Verification items for the finished model (mm, model axes). A direction names the side the tool comes from. Round coordinates to 2 decimals unless told otherwise and drop trailing zeros. Loops run counter-clockwise (first coordinate to the right, second up) from the corner with the lowest first, then second, coordinate; pieces in that order, holes last. Notation, with made-up numbers: (80.25, 78) -> (107.25, 78) arc R3 cw to (107.25, 82) -> close; hole circle Ø1 at (-29, 52.25). An arc over 180 degrees is marked (long way). Use a Markdown table: item, result. Add a question column.
```python
from build123d import *

# Parameters (mm, degrees)
CROQUIS1_W              = 144.567109546
CROQUIS1_H              = 113.391382114
SALIENTE_EXTRUIR1_DEPTH = 200
VACIADO2_T              = -10


with BuildPart() as part:
    # Croquis1 → Saliente-Extruir1 (new body)
    with BuildSketch(Plane.XY):
        Rectangle(CROQUIS1_W, CROQUIS1_H)
    extrude(amount=SALIENTE_EXTRUIR1_DEPTH)

    # Vaciado2
    vaciado2_openings = [part.faces().sort_by_distance(p)[0] for p in [
        (0, 0, 200),
    ]]
    offset(amount=VACIADO2_T, openings=vaciado2_openings, kind=Kind.INTERSECTION)


solid = part.part
```
1) Thickness scan on line 1 (X direction, y = -22.5, z = 135); line 2 (Y direction, x = -53.5, z = 21); line 3 (Z direction, x = -29.5, y = 3.5). Record the ranges inside material, lowest first.
2) Release check for a two-part mould opening along Y. For faces 1 (the face through (-1, 56.696, 99)), 2 (the face through (-62.284, -1, 104)), 3 (the face through (72.284, -1, 99)) record: released by +Y, released by -Y, zero draft, split by the parting line, or undercut.
3) Access from +Z, -Z, +X, -X, +Y, -Y to the whole of each face (thin tool, end or side, straight path). Record for faces 4 (the face through (-1, -56.696, 99)), 5 (the face through (-1, 1, 10)).
4) Go/stop test with a flat-tipped pin: pin 1 (5 mm diameter, centred on x = 41, y = -21, fed in from +Z). Record where the tip stops, or that it passes through.
5) Sectioned sample at C-C on x = 48. Enter the section's corners in (y, z).
6) Sectioned sample at B-B on y = 29.5. Enter the section's corners in (x, z), then the cut area to 3 significant figures.
7) Sectioned sample at A-A on z = 33. Enter the section's corners in (x, y).
Geometry results:
| question | item | result |
|---|---|---|
| 1 | line 1 | -72.28 to -62.28, 62.28 to 72.28 |
| 1 | line 2 | -56.7 to -46.7, 46.7 to 56.7 |
| 1 | line 3 | 0 to 10 |
| 2 | face 1 | released by +Y |
| 2 | face 2 | undercut |
| 2 | face 3 | zero draft |
| 3 | face 4 | +Z, -Z, +X, -X, -Y |
| 3 | face 5 | +Z |
| 4 | pin 1 | z = 10 |
| 5 | outline | (-56.7, 0) -> (56.7, 0) -> (56.7, 200) -> (46.7, 200) -> (46.7, 10) -> (-46.7, 10) -> (-46.7, 200) -> (-56.7, 200) -> close |
| 6 | outline | (-72.28, 0) -> (72.28, 0) -> (72.28, 200) -> (62.28, 200) -> (62.28, 10) -> (-62.28, 10) -> (-62.28, 200) -> (-72.28, 200) -> close |
| 6 | area | 5,250 mm^2 |
| 7 | outline | (-72.28, -56.7) -> (72.28, -56.7) -> (72.28, 56.7) -> (-72.28, 56.7) -> close; hole (-62.28, -46.7) -> (62.28, -46.7) -> (62.28, 46.7) -> (-62.28, 46.7) -> close |
